For this review, take the finished solid that the model builds, in its own axes (mm). A direction names the side the tool comes from. Coordinates: 2 decimals unless noted, no trailing zeros. Order: outer loops, then holes, each group sorted by start corner. A loop starts at its lowest first (then second) coordinate and runs counter-clockwise, first axis right, second up. Notation, with made-up numbers: (-19.5, 24.5) -> (-4.5, 24.5) arc R21 cw to (-4.5, 61.5) -> close; hole circle Ø6 at (-14, -30.75). An arc over 180 degrees is marked (long way). Write item = value, one per line. Start each with the question number.
1) Consider section B-B on x = 10.5. Give the boundary of the cut face in (y, z), and give its area (3 significant figures).
2) Consider section D-D on z = 10. Give the boundary of the cut face in (x, y).
3) Wall thickness on probe 1 along Z at (x, y) = (-10.5, -0.6); probe 2 along Y at (x, z) = (6.25, 9); probe 3 along X at (y, z) = (-1.5, -1): over which ranges is each line inside the solid? List them lowest first. Write a range as [from, to].
4) Machinability: for faces 5 (the face through (0, -3, -6.5)), 6 (the face through (4, -3, -3)), 7 (the face through (-12.5, -0.5, -0.2)), which of the approach directions +Z, -Z, +X, -X, +Y, -Y give a long, thin tool a straight path to every point of the face, cutting with its end or side? Answer none if there is none.
5) Draft analysis for pull direction Z (two halves, no side actions). For faces 1 (the face through (-4, -3, -3)), 2 (the face through (9.7, -0.5, -3.1)), 3 (the face through (-0.2, -0.5, -12)), 4 (the face through (0, -3, 1.5)), state which applies: +Z half, -Z half, draft (parallel to the pull), parting line (faces both ways), or undercut.
6) Insertion check: pin 1 Ø1.5 at (x, y) = (-1.5, -2.5) entering from -Z; pin 2 Ø2.5 at (y, z) = (-4, -2.5) entering from +X; pin 3 Ø8 at (x, z) = (-3, 6) entering from -Y. Each pin has a flat end and moves straight along its axis. Give the tip position at first contact, or say it passes through.
7) Consider section C-C on x = -1.25. Give the boundary of the cut face in (y, z), and give its area (3 significant figures).
8) Consider section A-A on z = -2.5. Give the boundary of the cut face in (x, y).
from build123d import *

# Parameters (mm, degrees)
F0_W     = 25
F0_H     = 24
F1_DEPTH = 1
F2_W     = 8
F2_H     = 8
F3_DEPTH = 5
F4_R     = 1
F5_DEPTH = 1.001


with BuildPart() as f1:
    # F0 (on Front) → F1 (new body)
    with BuildSketch(Plane.XZ):
        Rectangle(F0_W, F0_H)
    extrude(amount=F1_DEPTH)

    # F2 (on face) → F3 (join)
    with BuildSketch(Plane.XZ.offset(1)):
        with Locations((0, -2.5)):
            Rectangle(F2_W, F2_H)
    extrude(amount=F3_DEPTH)

    # F4 (on face) → F5 (cut, through all)
    with BuildSketch(Plane.XZ.offset(1)):
        with Locations((10.5, 10)):
            Circle(F4_R)
        with Locations((-10.5, 10)):
            Circle(F4_R)
        with Locations((-10.5, -2.5)):
            Circle(F4_R)
        with Locations((10.5, -2.5)):
            Circle(F4_R)
    extrude(amount=-F5_DEPTH, mode=Mode.SUBTRACT)


solid = f1.part
Answer sheet:
q1.outline = (-1, -12) -> (0, -12) -> (0, -3.5) -> (-1, -3.5) -> close; (-1, -1.5) -> (0, -1.5) -> (0, 9) -> (-1, 9) -> close; (-1, 11) -> (0, 11) -> (0, 12) -> (-1, 12) -> close
q1.area = 20.0 mm2
q2.outline = (-12.5, -1) -> (-11.5, -1) -> (-11.5, 0) -> (-12.5, 0) -> close; (-9.5, -1) -> (9.5, -1) -> (9.5, 0) -> (-9.5, 0) -> close; (11.5, -1) -> (12.5, -1) -> (12.5, 0) -> (11.5, 0) -> close
q3.probe_1 = [-12, -3.5], [-1.5, 9], [11, 12]
q3.probe_2 = [-1, 0]
q3.probe_3 = [-4, 4]
q4.face_5 = -Z, +X, -X, -Y
q4.face_6 = +Z, -Z, +X, -Y
q4.face_7 = +Z, -Z, -X, +Y, -Y
q5.face_1 = draft
q5.face_2 = undercut
q5.face_3 = -Z half
q5.face_4 = +Z half
q6.pin_1 = -6.5
q6.pin_2 = 4
q6.pin_3 = -1
q7.outline = (-6, -6.5) -> (-1, -6.5) -> (-1, -12) -> (0, -12) -> (0, 12) -> (-1, 12) -> (-1, 1.5) -> (-6, 1.5) -> close
q7.area = 64.0 mm2
q8.outline = (-12.5, -1) -> (-11.5, -1) -> (-11.5, 0) -> (-12.5, 0) -> close; (-9.5, -1) -> (-4, -1) -> (-4, -6) -> (4, -6) -> (4, -1) -> (9.5, -1) -> (9.5, 0) -> (-9.5, 0) -> close; (11.5, -1) -> (12.5, -1) -> (12.5, 0) -> (11.5, 0) -> close
